For this review, take the finished solid that the model builds, in its own axes (mm). A direction names the side the tool comes from. Round coordinates to 2 decimals unless told otherwise and drop trailing zeros. Write each loop counter-clockwise with the first axis right and the second up, starting at its lowest first coordinate (ties: lowest second). Pieces come first, ordered by that corner, then holes. Notation, with made-up numbers: M 56.25,86.5 L 110.25,86.5 A6 ccw 110.25,96.5 Z; hole C -30,43.25 d7. An arc over 180 degrees is marked long. One line per question, with ' | ' between items.
```python
from build123d import *

# Parameters (mm, degrees)
BOSS_EXTRUDE1_DEPTH = 55.8
BOSS_EXTRUDE2_DEPTH = 55.8
SKETCH5_W           = 1
SKETCH5_H           = 55.8
CUT_EXTRUDE3_DEPTH  = 1
LPATTERN1_COUNT     = 37
LPATTERN1_PITCH     = 2
SKETCH6_W           = 27
SKETCH6_H           = 3
BOSS_EXTRUDE3_DEPTH = 2


with BuildPart() as part:
    # Sketch1 → Boss-Extrude1 (new body)
    with BuildSketch(Plane(origin=(0, 0, 0), x_dir=(1, 0, 0), z_dir=(0, 1, 0))):
        Polygon((0, 0), (0, 80.15), (22, 80.15), (22, 83.15), (0, 83.15), (-5, 83.15), (-5, 0), align=None)
    extrude(amount=BOSS_EXTRUDE1_DEPTH)

    # Sketch2 → Boss-Extrude2 (add)
    with BuildSketch(Plane(origin=(0, 55.8, 0), x_dir=(1, 0, 0), z_dir=(0, 1, 0))):
        with BuildLine():
            Line((0, 80.15), (7.5, 80.15))
            ThreePointArc((7.5, 80.15), (3.126786079, 78.938689869), (0, 75.65))
            Line((0, 75.65), (0, 80.15))
        make_face()
    extrude(amount=-BOSS_EXTRUDE2_DEPTH)

    # Sketch5 → Cut-Extrude3 (cut)
    with BuildSketch(Plane(origin=(0, 0, 0), x_dir=(0, 0, -1), z_dir=(1, 0, 0))):
        with Locations((74.15, 27.9)):
            Rectangle(SKETCH5_W, SKETCH5_H)
    cut_extrude3 = extrude(amount=-CUT_EXTRUDE3_DEPTH, mode=Mode.SUBTRACT)

    # LPattern1: Cut-Extrude3 ×37
    with Locations(*[(0, 0, i * LPATTERN1_PITCH) for i in range(1, LPATTERN1_COUNT)]):
        add(cut_extrude3, mode=Mode.SUBTRACT)

    # Sketch6 → Boss-Extrude3 (add)
    with BuildSketch(Plane(origin=(0, 55.8, 0), x_dir=(1, 0, 0), z_dir=(0, 1, 0))):
        with Locations((8.5, 81.65)):
            Rectangle(SKETCH6_W, SKETCH6_H)
    extrude(amount=BOSS_EXTRUDE3_DEPTH)


solid = part.part
```
Item 1: Take a section at C-C (x = 4.25). Write out the cut boundary in (y, z).
Results:
outline: M 0,-83.15 L 57.8,-83.15 L 57.8,-80.15 L 55.8,-80.15 L 55.8,-79.5 L 0,-79.5 Z
Item 2: Machinability: for faces 1 (the face through (-3, 55.8, -41)), 2 (the face through (0, 28, -1)), 3 (the face through (8, 57.8, -82)), which of the approach directions +Z, -Z, +X, -X, +Y, -Y give a long, thin tool a straight path to every point of the face, cutting with its end or side? Answer none if there is none.
Results:
face 1: +Z, +X, -X, +Y | face 2: +Z, +X, +Y, -Y | face 3: +Z, -Z, +X, -X, +Y
Item 3: Take a section at A-A (x = -2). Write out the cut boundary in (y, z).
Results:
outline: M 0,-83.15 L 57.8,-83.15 L 57.8,-80.15 L 55.8,-80.15 L 55.8,0 L 0,0 Z
Item 4: To check wall thickness, follow line 1 along Z through (x, y) = (7, 14.5); line 2 along X through (y, z) = (24, -16); line 3 along Z through (x, y) = (20.25, 36). State the ranges of each line that lie inside material, in increasing order. Write a range as from..to.
Results:
line 1: -83.15..-80.14 | line 2: -5..-1 | line 3: -83.15..-80.15
Item 5: Insertion check: pin 1 Ø0.5 at (y, z) = (25.5, -12.5) entering from +X. The pin has a flat end and moves straight along its axis. Give the tip position at first contact, or say it passes through.
Results:
pin 1: x = 0
Item 6: Take a section at B-B (x = 14.5). Write out the cut boundary in (y, z).
Results:
outline: M 0,-83.15 L 57.8,-83.15 L 57.8,-80.15 L 0,-80.15 Z
